```python
from build123d import *

# Parameters (mm, degrees)
SKETCH_1_R          = 1
EXTRUDE_1_DEPTH     = 9
SKETCH_2_W          = 7.4
SKETCH_2_H          = 10
CUT_EXTRUDE_1_DEPTH = 9
SKETCH_3_W          = 0.8
SKETCH_3_H          = 15.035626068
CUT_EXTRUDE_2_DEPTH = 9
FILLET_2_R          = 3.7
SKETCH_4_W          = 7.4
SKETCH_4_H          = 2.039607805
CUT_EXTRUDE_3_DEPTH = 9
SKETCH_5_R          = 1.5
CUT_EXTRUDE_4_DEPTH = 9
FILLET_3_R          = 0.8


# Some blends are built 0.0001 mm under size
with BuildPart() as part:
    # 草图1 → 凸台-拉伸1 (new body)
    with BuildSketch(Plane.XY):
        with BuildLine():
            Line((3, 0), (5.196152423, 0))
            ThreePointArc((5.196152423, 0), (7.794228634, -1.5), (7.794228634, -4.5))
            ThreePointArc((7.794228634, -4.5), (4.842298019, -7.586313327), (0.8, -8.964373932))
            Line((0.8, -8.964373932), (0.8, -24))
            Line((0.8, -24), (0, -24))
            Line((0, -24), (0, -3))
            ThreePointArc((0, -3), (0.878679656, -0.878679656), (3, 0))
        make_face()
        with Locations((4.5, -3)):
            Circle(SKETCH_1_R, mode=Mode.SUBTRACT)
    extrude(amount=EXTRUDE_1_DEPTH)

    # 草图2 → 切除-拉伸1 (cut)
    with BuildSketch(Plane(origin=(0.8, 0, 0), x_dir=(0, 0, -1), z_dir=(1, 0, 0))):
        with Locations((-4.5, -3.964373932)):
            Rectangle(SKETCH_2_W, SKETCH_2_H)
    extrude(amount=CUT_EXTRUDE_1_DEPTH, mode=Mode.SUBTRACT)

    # 草图3 → 切除-拉伸2 (cut)
    with BuildSketch(Plane(origin=(0.8, 0, 0), x_dir=(0, 0, -1), z_dir=(1, 0, 0))):
        with Locations((-8.6, -16.482186966)):
            Rectangle(SKETCH_3_W, SKETCH_3_H)
        with Locations((-0.4, -16.482186966)):
            Rectangle(SKETCH_3_W, SKETCH_3_H)
    extrude(amount=-CUT_EXTRUDE_2_DEPTH, mode=Mode.SUBTRACT)

    # 圆角2
    fillet_2_edges = [part.edges().sort_by_distance(p)[0] for p in [
        (0.4, -24, 0.8),
        (0.4, -24, 8.2),
    ]]
    fillet(fillet_2_edges, radius=FILLET_2_R - 0.0001)  # a hair under: the kernel refuses the full size

    # 草图4 → 切除-拉伸3 (cut)
    with BuildSketch(Plane.ZY):
        with Locations((4.5, -1.980196097)):
            Rectangle(SKETCH_4_W, SKETCH_4_H)
    extrude(amount=-CUT_EXTRUDE_3_DEPTH, mode=Mode.SUBTRACT)

    # 草图5 → 切除-拉伸4 (cut)
    with BuildSketch(Plane(origin=(0.8, 0, 0), x_dir=(0, 0, -1), z_dir=(1, 0, 0))):
        with Locations(Location((-4.5, -8.3, 0), (0, 0, 90))):
            Circle(SKETCH_5_R)
        with Locations(Location((-4.5, -19.5, 0), (0, 0, 90))):
            Circle(SKETCH_5_R)
    extrude(amount=-CUT_EXTRUDE_4_DEPTH, mode=Mode.SUBTRACT)

    # 圆角3
    # the kernel refuses this fillet: 0.8 mm, written as the material it adds along each edge
    with BuildSketch(Plane(origin=(0.8, -8.964373932, 0.8), x_dir=(0, -1, 0), z_dir=(-1, 0, 0))) as fillet_3_piece_1:
        with BuildLine():
            CenterArc((FILLET_3_R, -FILLET_3_R), FILLET_3_R, 90, 90)
            Line((0, -FILLET_3_R), (0, 0))
            Line((0, 0), (FILLET_3_R, 0))
        make_face()
    extrude(amount=0.8)
    with BuildSketch(Plane(origin=(0.8, -8.964373932, 8.2), x_dir=(0, -1, 0), z_dir=(-1, 0, 0))) as fillet_3_piece_2:
        with BuildLine():
            CenterArc((FILLET_3_R, FILLET_3_R), FILLET_3_R, 180, 90)
            Line((0, FILLET_3_R), (0, 0))
            Line((0, 0), (FILLET_3_R, 0))
        make_face()
    extrude(amount=0.8)
    with BuildSketch(Plane(origin=(-2, -3, 0.8), x_dir=(0, 0, 1), z_dir=(1, 0, 0))) as fillet_3_piece_3_section:
        with BuildLine():
            CenterArc((FILLET_3_R, -FILLET_3_R), FILLET_3_R, 90, 90)
            Line((0, -FILLET_3_R), (0, 0))
            Line((0, 0), (FILLET_3_R, 0))
        make_face()
    fillet_3_piece_3 = extrude(amount=2.8, mode=Mode.PRIVATE)
    fillet_3_piece_3 = fillet_3_piece_3 & Plane(origin=(3, -3, 0.979954946), x_dir=(-1, 0, 0), z_dir=(0, 0, -1)) * Cylinder(3, 9, mode=Mode.PRIVATE)
    add(fillet_3_piece_3)
    with BuildSketch(Plane(origin=(-2, -3, 8.2), x_dir=(0, 0, -1), z_dir=(1, 0, 0))) as fillet_3_piece_4_section:
        with BuildLine():
            CenterArc((FILLET_3_R, FILLET_3_R), FILLET_3_R, 180, 90)
            Line((0, FILLET_3_R), (0, 0))
            Line((0, 0), (FILLET_3_R, 0))
        make_face()
    fillet_3_piece_4 = extrude(amount=2.8, mode=Mode.PRIVATE)
    fillet_3_piece_4 = fillet_3_piece_4 & Plane(origin=(3, -3, 8.020045054), x_dir=(-1, 0, 0), z_dir=(0, 0, -1)) * Cylinder(3, 9, mode=Mode.PRIVATE)
    add(fillet_3_piece_4)


solid = part.part
```
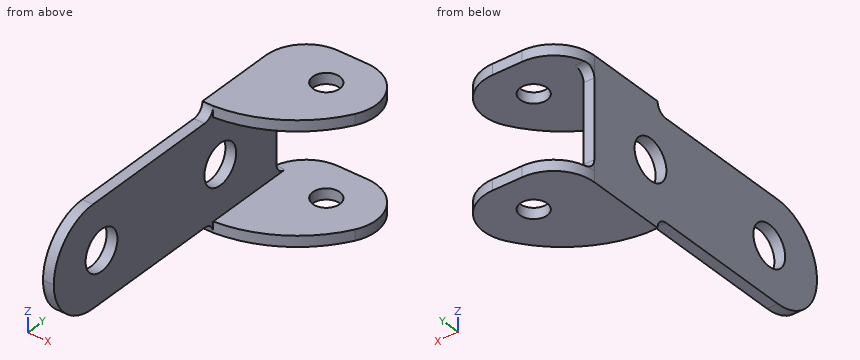
For this review, take the finished solid that the model builds, in its own axes (mm). Coordinates: 2 decimals unless noted, no trailing zeros. Order: outer loops, then holes, each group sorted by start corner. A loop starts at its lowest first (then second) coordinate and runs counter-clockwise, first axis right, second up. Notation, with made-up numbers: (34.25, 20.25) - (61.25, 20.25) arc R29 cw to (61.25, 43.25) - close; hole circle Ø4 at (-37.75, 39.25). An arc over 180 degrees is marked (long way). Answer as a JSON object with one key per item and string values. Group by question number.
1. We need section D-D on z = 7.75. State the section outline as (x, y) points.
2. Clearance check with a flat-ended pin moving along its axis: P1, Ø0.6, axis at x = 0.5, z = 3.5, coming from the +Y side. State where the tip first meets the part, or that it passes through.
3. We need section C-C on x = 4.5. State the section outline as (y, z) points, then the cut area to 3 significant figures.
4. We need section A-A on y = -19.5. State the section outline as (x, z) points.
5. We need section B-B on x = 1.5. State the section outline as (y, z) points.
6. For probe 1 along Z at (x, y) = (0.35, -8.3); probe 2 along Z at (x, y) = (2.5, -4.5); probe 3 along X at (y, z) = (-19, 2.5), list the stretches that pass through material, from the lowest coordinate up.
Final values:
{
 "1": {"outline": "(0, -22.07) - (0.8, -22.07) - (0.8, -2.92) - (0, -2.92) arc R3 ccw to (0, -3) - close"},
 "2": {"P1": "y = -3"},
 "3": {"outline": "(-7.79, 0) - (-4, 0) - (-4, 0.8) - (-7.79, 0.8) - close; (-7.79, 8.2) - (-4, 8.2) - (-4, 9) - (-7.79, 9) - close; (-2, 0) - (0, 0) - (0, 0.8) - (-2, 0.8) - close; (-2, 8.2) - (0, 8.2) - (0, 9) - (-2, 9) - close", "area": "9.27 mm²"},
 "4": {"outline": "(0, 0.8) - (0.8, 0.8) - (0.8, 3) - (0, 3) - close; (0, 6) - (0.8, 6) - (0.8, 8.2) - (0, 8.2) - close"},
 "5": {"outline": "(-8.87, 0) - (-0.4, 0) - (-0.4, 0.8) - (-8.87, 0.8) - close; (-8.87, 8.2) - (-0.4, 8.2) - (-0.4, 9) - (-8.87, 9) - close"},
 "6": {"probe 1": "0 to 3, 6 to 9", "probe 2": "0 to 0.8, 8.2 to 9", "probe 3": "0 to 0.8"}
}
